```python
from build123d import *

# Parameters (mm, degrees)
F1_DEPTH = 50.8
F3_R     = 4.7625
F4_DEPTH = 9.525
F6_R     = 4.7625
F7_DEPTH = 9.525
F8_R     = 4.7625
F9_DEPTH = 25.4


with BuildPart() as f1:
    # F0 (on Top) → F1 (new body)
    with BuildSketch(Plane.XY):
        Polygon((-355.6, 0), (-355.6, -9.525), (355.6, -9.525), (355.6, 0), (406.4, 0), (406.4, 9.525), (-406.4, 9.525), (-406.4, 0), align=None)
    extrude(amount=F1_DEPTH)

    # F3 (on offset) → F4 (join)
    with BuildSketch(Plane.YZ.offset(406.4)):
        with Locations((0, 25.4)):
            Circle(F3_R)
    extrude(amount=F4_DEPTH)

    # F6 (on offset) → F7 (join)
    with BuildSketch(Plane.YZ.offset(-406.4)):
        with Locations((0, 25.418339)):
            Circle(F6_R)
    extrude(amount=-F7_DEPTH)

    # F8 (on Front) → F9 (cut)
    with BuildSketch(Plane.XZ):
        with Locations((-396.875, 25.4)):
            Circle(F8_R)
        with Locations((396.875, 25.4)):
            Circle(F8_R)
    extrude(amount=-F9_DEPTH, mode=Mode.SUBTRACT)


solid = f1.part
```
Source: CAD feature listing. Evaluate the final solid. Frame: model axes, mm. Give positions to 0.01 mm unless a question says otherwise; leave off trailing zeros. Write each loop counter-clockwise with the first axis right and the second up, starting at its lowest first coordinate (ties: lowest second). Pieces come first, ordered by that corner, then holes. Notation, with made-up numbers: (26, -7) - (49, -7) arc R26 ccw to (49, 30) - close; hole circle Ø1 at (75.25, 31). An arc over 180 degrees is marked (long way). One line per item, written item: value. Start each with the question number.
Q1. Material intervals for probe 1 along X at (y, z) = (-7, 15.5); probe 2 along X at (y, z) = (4.25, 35.5); probe 3 along X at (y, z) = (0.75, 29) (3 decimals), sorted ascending. Write a range as from..to.
Q2. Section query A-A, the plane x = -366. Return the cut outline in (y, z) (3 decimals).
Q3. First-contact query: pin 1 Ø5 at (y, z) = (5.5, 22) entering from +X (3 decimals); pin 2 Ø8 at (y, z) = (0.5, 40) entering from -X; pin 3 Ø8.5 at (x, z) = (396.875, 25.4) entering from +Y; pin 4 Ø15 at (x, z) = (-392.5, 26) entering from -Y. Flat tips, straight axial feed; report the tip coordinate or a pass-through.
Answer:
1. probe 1: x = -355.6..355.6
1. probe 2: x = -406.4..406.4
1. probe 3: x = -415.925..-399.993, -393.757..393.757, 399.993..415.925
2. outline: (0, 0) - (9.525, 0) - (9.525, 50.8) - (0, 50.8) - close
3. pin 1: stops at x = 415.925
3. pin 2: stops at x = -406.4
3. pin 3: passes through
3. pin 4: stops at y = 0
